Can you work these out from the model? Positions are in its coordinate system, mm. A direction names the side the tool comes from. Give positions to 0.01 mm unless a question says otherwise; leave off trailing zeros. Loops run counter-clockwise (first coordinate to the right, second up) from the corner with the lowest first, then second, coordinate; pieces in that order, holes last. Notation, with made-up numbers: M -29.5,61.5 L 1.5,61.5 A27 ccw 1.5,91.5 Z; hole C 38,-36.75 d11. An arc over 180 degrees is marked long. Put each result on its own line as item: value. Start each with the question number.
1) Imagine slicing it at D-D (z = 1199.5). Write out the boundary of the cut face in (x, y).
2) For P1, Ø8, axis at x = -597.5, y = 18992, coming from the +Z side; P2, Ø5, axis at y = 18904.5, z = 901, coming from the +X side; P3, Ø10, axis at x = -9, z = 1460.5, coming from the +Y side, each with a flat end and sliding along its axis, tell me the tip position at first contact or that it passes through.
3) Imagine slicing it at B-B (y = 18950). Write out the boundary of the cut face in (x, z), then the cut area to 3 significant figures.
4) If we mould it in two halves opening along X, with no side actions, what happens to faces 1 (the flat face through (339.439, 18950.7, 35.537)), 2 (the flat face through (-2, 18948, 900)), 3 (the flat face through (171.246, 18949.3, 467.35)), 4 (the flat face through (-328.199, 18950.7, 61.056))? For each: +X half, -X half, draft (parallel to the pull), parting line (faces both ways), or undercut.
5) Imagine slicing it at A-A (z = 374.5). Write out the boundary of the cut face in (x, y), then the cut area to 3 significant figures.
6) Please list where these lines run through material, in increasing order: line 1 along Z through (x, y) = (-413.5, 18979); line 2 along Y through (x, z) = (653, 1492); line 3 along Z through (x, y) = (-76, 18788). Write a range as from..to.
7) For faces 5 (the flat face through (-164.875, 18949.3, 480.11)), 6 (the flat face through (591, 18949, 1414.222)), 7 (the cylindrical face through (-119.035, 19041.273, 1289.23)), which set-ups out of +Z, -Z, +X, -X, +Y, -Y let a thin tool reach every point of the face, with its end or its side?
8) Imagine slicing it at C-C (x = -103). Write out the boundary of the cut face in (y, z), then the cut area to 3 significant figures.
from build123d import *

# Parameters (mm, degrees)
BOX002_W               = 100
BOX002_H               = 100
BOX002_DEPTH           = 1000
BOX002_PLACEMENT_ANGLE = 165
BOX001_W               = 100
BOX001_H               = 100
BOX001_DEPTH           = 1000
BOX001_PLACEMENT_ANGLE = 195
CYLINDER004_R          = 150
CYLINDER004_DEPTH      = 900
BOX003_W               = 100
BOX003_H               = 100
BOX003_DEPTH           = 2000


with BuildPart() as cube002:
    # Box002 → Box002 (new body)
    with BuildSketch(Plane.XY):
        with Locations((50, 50)):
            Rectangle(BOX002_W, BOX002_H)
    extrude(amount=BOX002_DEPTH)


with BuildPart() as cube002_1:
    # Box002 placement: moved
    add(cube002.part.moved(Location((-21.759997, -50, 1014.222118))).rotate(Axis((-21.759997, -50, 1014.222118), (0, -1, 0)), BOX002_PLACEMENT_ANGLE))


with BuildPart() as cube001:
    # Box001 → Box001 (new body)
    with BuildSketch(Plane.XY):
        with Locations((50, 50)):
            Rectangle(BOX001_W, BOX001_H)
    extrude(amount=BOX001_DEPTH)


with BuildPart() as cube001_1:
    # Box001 placement: moved
    add(cube001.part.moved(Location((128.240003, -50, 1014.222118))).rotate(Axis((128.240003, -50, 1014.222118), (0, -1, 0)), BOX001_PLACEMENT_ANGLE))


with BuildPart() as sphere003:
    # Sphere003 → Sphere003 (revolve)
    with BuildSketch(Plane(origin=(0, 0, 1800), x_dir=(1, 0, 0), z_dir=(0, -1, 0))):
        with BuildLine():
            ThreePointArc((0, -200), (200, 0), (0, 200))
            Line((0, 200), (0, -200))
        make_face()
    revolve(axis=Axis((0, 0, 1800), (0, 0, 1)))


with BuildPart() as cylinder004:
    # Cylinder004 → Cylinder004 (new body)
    with BuildSketch(Plane(origin=(0, 0, 1800), x_dir=(1, 0, 0), z_dir=(0, 0, -1))):
        Circle(CYLINDER004_R)
    extrude(amount=CYLINDER004_DEPTH)


with BuildPart() as fusion001:
    # Box003 → Box003 (new body)
    with BuildSketch(Plane(origin=(1028.240003, -50, 1414.222118), x_dir=(0, 0, 1), z_dir=(-1, 0, 0))):
        with Locations((50, 50)):
            Rectangle(BOX003_W, BOX003_H)
    extrude(amount=BOX003_DEPTH)

    # Fusion001: union Cube002, Cube001, Sphere003, Cylinder004
    add(cube002_1.part)
    add(cube001_1.part)
    add(sphere003.part)
    add(cylinder004.part)


with BuildPart() as fusion001_1:
    # Fusion001 placement: moved
    add(fusion001.part.moved(Location((0, 18950, 0))))


solid = fusion001_1.part
Recorded:
1. outline: C 0,18950 d300
2. P1: z = 1514.22
2. P2: x = 159.25
2. P3: y = 19099.95
3. outline: M -971.76,1414.22 L -150,1414.22 L -150,921.99 L -377.17,74.18 L -280.58,48.3 L -52.37,900 L 55.32,900 L 290.47,22.41 L 387.06,48.3 L 150,933.01 L 150,1414.22 L 1028.24,1414.22 L 1028.24,1514.22 L 150,1514.22 L 150,1667.71 A200 ccw long -150,1667.71 L -150,1514.22 L -971.76,1514.22 Z
3. area: 688,000 mm²
4. face 1: +X half
4. face 2: undercut
4. face 3: undercut
4. face 4: -X half
5. outline: M -296.7,18900 L -193.17,18900 L -193.17,19000 L -296.7,19000 Z; M 196.13,18900 L 299.65,18900 L 299.65,19000 L 196.13,19000 Z
5. area: 20,700 mm²
6. line 1: 1414.22..1514.22
6. line 2: 18900..19000
6. line 3: 1710.67..1889.33
7. face 5: -Z, +Y, -Y
7. face 6: +X, +Y, -Y
7. face 7: none
8. outline: M 18840.95,900 L 18900,900 L 18900,711.03 L 19000,711.03 L 19000,900 L 19059.05,900 L 19059.05,1667.71 A171.44 ccw long 18840.95,1667.71 Z
8. area: 273,000 mm²
